```python
from build123d import *

# Parameters (mm, degrees)
F0_R     = 1.397
F0_R_2   = 3.81
F0_R_3   = 1.651
F0_R_4   = 1.7145
F1_DEPTH = 2.286


with BuildPart() as f1:
    # F0 (on Top) → F1 (new body)
    with BuildSketch(Plane.XY):
        with BuildLine():
            ThreePointArc((1.919111, -21.504537), (15.930501, -14.572139), (21.59, 0))
            ThreePointArc((21.59, 0), (15.930501, 14.572139), (1.919111, 21.504537))
            ThreePointArc((1.919111, 21.504537), (-21.59, 0), (1.919111, -21.504537))
        make_face()
        with Locations((-7.493, 0)):
            Circle(F0_R, mode=Mode.SUBTRACT)
        Circle(F0_R_2, mode=Mode.SUBTRACT)
        with Locations((7.493, 0)):
            Circle(F0_R, mode=Mode.SUBTRACT)
        with BuildLine():
            ThreePointArc((1.919111, 21.504537), (15.930501, 14.572139), (21.59, 0))
            ThreePointArc((21.59, 0), (15.930501, -14.572139), (1.919111, -21.504537))
            Line((1.919111, -21.504537), (86.966778, -13.9147))
            ThreePointArc((86.966778, -13.9147), (71.755, 0), (86.966778, 13.9147))
            Line((86.966778, 13.9147), (1.919111, 21.504537))
        make_face()
        with Locations((27.94, -11.532094)):
            Circle(F0_R_3, mode=Mode.SUBTRACT)
        with Locations((65.405, -8.188637)):
            Circle(F0_R_3, mode=Mode.SUBTRACT)
        with Locations((27.94, 0)):
            Circle(F0_R_3, mode=Mode.SUBTRACT)
        with Locations((27.94, 11.532094)):
            Circle(F0_R_3, mode=Mode.SUBTRACT)
        with Locations((65.405, 0)):
            Circle(F0_R_3, mode=Mode.SUBTRACT)
        with Locations((65.405, 8.188637)):
            Circle(F0_R_3, mode=Mode.SUBTRACT)
        with BuildLine():
            ThreePointArc((99.695, 0), (96.032971, 9.429031), (86.966778, 13.9147))
            ThreePointArc((86.966778, 13.9147), (71.755, 0), (86.966778, -13.9147))
            ThreePointArc((86.966778, -13.9147), (96.032971, -9.429031), (99.695, 0))
        make_face()
        with Locations((85.725, 0)):
            Circle(F0_R_4, mode=Mode.SUBTRACT)
    extrude(amount=F1_DEPTH)


solid = f1.part
```
The listing builds one solid part. Answer for the finished solid, in the listing's coordinates (mm). Coordinates: 2 decimals unless noted, no trailing zeros. Loops run counter-clockwise (first coordinate to the right, second up) from the corner with the lowest first, then second, coordinate; pieces in that order, holes last. Notation, with made-up numbers: M -28.5,73.25 L -19.5,73.25 A37 ccw -19.5,112.25 Z; hole C -38.5,16 d2. An arc over 180 degrees is marked long. Answer as CSV lines item,"result". Start each with the question number.
(1) The part is cut by section C-C (x = 27.94). Give the vertices of the cut face in (y, z).
(2) The part is cut by section D-D (y = -18). Give the vertices of the cut face in (x, z).
(3) The part is cut by section A-A (x = 0). Give the vertices of the cut face in (y, z).
(4) Find the intervals of material crossed by L1, parallel to Y at x = 27.94, z = 0.5; L2, parallel to X at y = -2, z = 0.35; L3, parallel to Y at x = 8.5, z = 0.7, in increasing order. Write a range as [from, to].
(5) The part is cut by section B-B (z = 0.5). State how many separate pieces and enclosed holes the cut face has, and give its area (3 significant figures).
(6) The mould has two halves that part along X. Classify faces 1 (the flat face through (38, 0, 2.286)), 2 (the flat face through (45.038, 17.656, 1.127)), 3 (the cylindrical face through (66.93, 7.56, 1.13)), 4 (the cylindrical face through (-0.83, -3.72, 1.13)): pulls with the +X half, pulls with the -X half, needs draft (parallel to the pull), parting line crosses it, or undercut.
Determined:
1,outline,"M -19.18,0 L -13.18,0 L -13.18,2.29 L -19.18,2.29 Z; M -9.88,0 L -1.65,0 L -1.65,2.29 L -9.88,2.29 Z; M 1.65,0 L 9.88,0 L 9.88,2.29 L 1.65,2.29 Z; M 13.18,0 L 19.18,0 L 19.18,2.29 L 13.18,2.29 Z"
2,outline,"M -11.92,0 L 41.19,0 L 41.19,2.29 L -11.92,2.29 Z"
3,outline,"M -21.59,0 L -3.81,0 L -3.81,2.29 L -21.59,2.29 Z; M 3.81,0 L 21.59,0 L 21.59,2.29 L 3.81,2.29 Z"
4,L1,"[-19.18, -13.18], [-9.88, -1.65], [1.65, 9.88], [13.18, 19.18]"
4,L2,"[-21.5, -3.24], [3.24, 99.55]"
4,L3,"[-20.92, -0.97], [0.97, 20.92]"
5,separate pieces,"1"
5,enclosed holes,"10"
5,area,"3,980 mm2"
6,face 1,"needs draft"
6,face 2,"pulls with the +X half"
6,face 3,"undercut"
6,face 4,"undercut"
